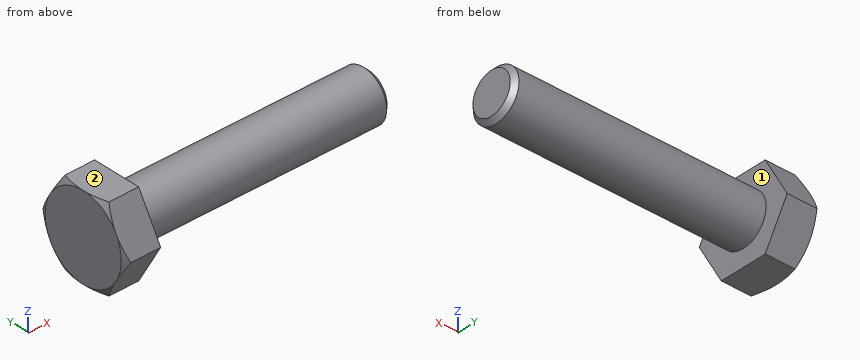
```python
from build123d import *

# Parameters (mm, degrees)
BASEHEAD_DEPTH = 4


with BuildPart() as part:
    # Sketch1 → BaseHead (new body)
    with BuildSketch(Plane(origin=(0, 0, 0), x_dir=(0, 0, -1), z_dir=(1, 0, 0))):
        Polygon((5, 2.886751346), (5, -2.886751346), (0, -5.773502692), (-5, -2.886751346), (-5, 2.886751346), (0, 5.773502692), align=None)
    extrude(amount=BASEHEAD_DEPTH)

    # BodySke → BaseBody (revolve)
    with BuildSketch(Plane.XY):
        Polygon((0, 0), (34, 0), (34, 2.4455), (33.4455, 3), (0, 3), align=None)
    revolve(axis=Axis((0, 0, 0), (1, 0, 0)))

    # Sketch3 → HeadChamfer (revolve, cut)
    with BuildSketch(Plane.XY):
        Polygon((0, 5), (3.333333333, 10.773502692), (3.333333333, 15.773502692), (-10, 15.773502692), (-10, 5), align=None)
    revolve(axis=Axis((0, 0, 0), (1, 0, 0)), mode=Mode.SUBTRACT)


solid = part.part
```
Geometry: final body of the model. Coordinates: model frame, mm. Face numbers are marked on the shaded views. A direction names the side the tool comes from. Give positions to 0.01 mm unless a question says otherwise; leave off trailing zeros. Loops run counter-clockwise (first coordinate to the right, second up) from the corner with the lowest first, then second, coordinate; pieces in that order, holes last. Notation, with made-up numbers: (58.5, -8.75) -> (87.5, -8.75) arc R32 cw to (87.5, 19.25) -> close; hole circle Ø3 at (-0.5, 84). An arc over 180 degrees is marked (long way). Return JSON: item names as keys, results as strings.
Item 1: Section A-A, the plane x = 24. Output: boundary loops of the cut face in (y, z), plus the area to 3 significant figures.
Filled in:
{"outline": "circle Ø6 at (0, 0)", "area": "28.3 mm^2"}
Item 2: Access query for the marked faces 1 and 2. Directions: +Z, -Z, +X, -X, +Y, -Y. A direction counts if a zero-diameter tool reaches every point of the face in a straight line with its end or side. Return the directions, or none.
Filled in:
{"face 1": "+X", "face 2": "+Z, +X, -X, +Y, -Y"}
Item 3: Pin query (flat end, axial travel): P1, Ø1.5, axis at x = 30, z = -1.5, coming from the +Y side; P2, Ø1, axis at x = 26, z = -2.5, coming from the -Y side; P3, Ø6, axis at x = 9, y = -0.5, coming from the -Z side. Return the tip coordinate at first contact, or that it passes through.
Filled in:
{"P1": "y = 2.9", "P2": "y = -2.24", "P3": "z = -3"}
Item 4: Line query: line 1 (X direction, y = 2, z = -2.5); line 2 (Z direction, x = 32, y = 0); line 3 (Z direction, x = 19.5, y = -1.5). Output: solid intervals per line, ascending.
Filled in:
{"line 1": "0 to 4", "line 2": "-3 to 3", "line 3": "-2.6 to 2.6"}
